```python
from build123d import *

# Parameters (mm, degrees)
SKETCH1_W           = 355.6
SKETCH1_H           = 762
BOSS_EXTRUDE1_DEPTH = 6.35
FILLET1_R           = 228.6
SKETCH3_R           = 95.25
CUT_EXTRUDE1_DEPTH  = 421.492761531
SKETCH2_R           = 3.3734375
CUT_EXTRUDE2_DEPTH  = 421.492761531
FILLET2_R           = 2.54


with BuildPart() as part:
    # Sketch1 → Boss-Extrude1 (new body)
    with BuildSketch(Plane.XY):
        Rectangle(SKETCH1_W, SKETCH1_H)
    extrude(amount=BOSS_EXTRUDE1_DEPTH)

    # Fillet1
    fillet1_edges = [part.edges().sort_by_distance(p)[0] for p in [
        (-177.8, 381, 3.175),
    ]]
    fillet(fillet1_edges, radius=FILLET1_R)

    # Sketch3 → Cut-Extrude1 (cut, through all)
    with BuildSketch(Plane.XY.offset(6.35)):
        with Locations((-177.8, -101.6)):
            Circle(SKETCH3_R)
    extrude(amount=-CUT_EXTRUDE1_DEPTH, mode=Mode.SUBTRACT)

    # Sketch2 → Cut-Extrude2 (cut, through all)
    with BuildSketch(Plane.XY.offset(6.35)):
        with Locations((146.05, 228.6)):
            Circle(SKETCH2_R)
        with Locations((38.1, 88.9)):
            Circle(SKETCH2_R)
        with Locations((-127, 88.9)):
            Circle(SKETCH2_R)
        with Locations((146.05, -190.5)):
            Circle(SKETCH2_R)
        with Locations((38.1, -330.2)):
            Circle(SKETCH2_R)
        with Locations((-127, -330.2)):
            Circle(SKETCH2_R)
    extrude(amount=-CUT_EXTRUDE2_DEPTH, mode=Mode.SUBTRACT)

    # Fillet2
    fillet2_edges = [part.edges().sort_by_distance(p)[0] for p in [
        (-177.8, -6.35, 3.175),
        (-177.8, -196.85, 3.175),
        (177.8, -381, 3.175),
        (-177.8, -381, 3.175),
        (177.8, 381, 3.175),
    ]]
    fillet(fillet2_edges, radius=FILLET2_R)


solid = part.part
```
Could you check a few things on this model? Use its own coordinates, in mm. Give positions to 0.01 mm unless a question says otherwise; leave off trailing zeros. Loops run counter-clockwise (first coordinate to the right, second up) from the corner with the lowest first, then second, coordinate; pieces in that order, holes last. Notation, with made-up numbers: (67.25, 15) - (119.25, 15) arc R9 cw to (119.25, 19) - close; hole circle Ø2 at (11.25, 7.5). An arc over 180 degrees is marked (long way). Answer in a Markdown table with one row per item. Add a question column.
Q1. If we section it at A-A (z = 3): List the corners of the cut face in (x, y) for me.
Q2. For pin 1 (8 mm diameter, centred on x = 146.05, y = -190.5, fed in from +Z), with a flat end and sliding along its axis, tell me the tip position at first contact or that it passes through.
Q3. If we section it at B-B (y = -101.6): List the corners of the cut face in (x, z) for me.
Q4. We'd pull the mould along Y, two halves only. Please class faces 1 (the face through (-112.61, 312.26, 3.22)), 2 (the face through (-82.572, -103.66, 3.219)), 3 (the face through (-2, 5, 6.35)): +Y half, -Y half, draft (parallel to the pull), parting line (faces both ways), or undercut.
Q5. Please list where these lines run through material, in increasing order: L1, parallel to Y at x = 146.5, z = 0.75; L2, parallel to X at y = -330.2, z = 1.75; L3, parallel to Y at x = 38.1, z = 4.5. Write a range as from..to.
The answers:
| question | item | result |
|---|---|---|
| 1 | outline | (-177.8, -378.46) arc R2.54 ccw to (-175.26, -381) - (175.26, -381) arc R2.54 ccw to (177.8, -378.46) - (177.8, 378.46) arc R2.54 ccw to (175.26, 381) - (50.8, 381) arc R228.6 ccw to (-177.8, 152.4) - (-177.8, -3.84) arc R2.54 ccw to (-175.33, -6.38) arc R95.25 cw to (-175.33, -196.82) arc R2.54 ccw to (-177.8, -199.36) - close; hole circle Ø6.75 at (-127, -330.2); hole circle Ø6.75 at (-127, 88.9); hole circle Ø6.75 at (38.1, -330.2); hole circle Ø6.75 at (38.1, 88.9); hole circle Ø6.75 at (146.05, -190.5); hole circle Ø6.75 at (146.05, 228.6) |
| 2 | pin 1 | stops at z = 6.35 |
| 3 | outline | (-82.55, 0) - (177.8, 0) - (177.8, 6.35) - (-82.55, 6.35) - close |
| 4 | face 1 | +Y half |
| 4 | face 2 | undercut |
| 4 | face 3 | draft |
| 5 | L1 | y = -381..-193.84, -187.16..225.26, 231.94..381 |
| 5 | L2 | x = -177.8..-130.37, -123.63..34.73, 41.47..177.8 |
| 5 | L3 | y = -381..-333.57, -326.83..85.53, 92.27..380.65 |
